from build123d import *

# Parameters (mm, degrees)
SKETCH2_W           = 5
SKETCH2_H           = 5.6
SKETCH2_R           = 1.5
BOSS_EXTRUDE1_DEPTH = 3
SKETCH5_W           = 5
SKETCH5_H           = 8
BOSS_EXTRUDE4_DEPTH = 3
BOSS_EXTRUDE5_DEPTH = 5
FILLET3_R           = 1


with BuildPart() as part:
    # Sketch2 → Boss-Extrude1 (new body)
    # profile 1 of 3: a face of its own
    with BuildSketch(Plane.XY):
        with Locations((-5, 0)):
            Rectangle(SKETCH2_W, SKETCH2_H)
        with Locations((-5, 0)):
            Circle(SKETCH2_R, mode=Mode.SUBTRACT)
    # profile 2 of 3: a face of its own
    with BuildSketch(Plane.XY):
        Rectangle(SKETCH2_W, SKETCH2_H)
    # profile 3 of 3: a face of its own
    with BuildSketch(Plane.XY):
        with Locations((5, 0)):
            Rectangle(SKETCH2_W, SKETCH2_H)
        with Locations((5, 0)):
            Circle(SKETCH2_R, mode=Mode.SUBTRACT)
    extrude(amount=BOSS_EXTRUDE1_DEPTH)

    # Sketch5 → Boss-Extrude4 (add)
    with BuildSketch(Plane.XY.offset(3)):
        with Locations((0, 6.8)):
            Rectangle(SKETCH5_W, SKETCH5_H)
    extrude(amount=-BOSS_EXTRUDE4_DEPTH)

    # Sketch6 → Boss-Extrude5 (add)
    with BuildSketch(Plane(origin=(2.5, 0, 0), x_dir=(0, 0, -1), z_dir=(1, 0, 0))):
        Polygon((0, 5.8), (11, 11.8), (11, 15.8), (-3, 12.8), (-3, 10.8), (0, 10.8), align=None)
    extrude(amount=-BOSS_EXTRUDE5_DEPTH)

    # Fillet3
    fillet3_edges = [part.edges().sort_by_distance(p)[0] for p in [
        (0, -2.8, 3),
        (-7.5, -2.8, 1.5),
        (-7.5, 2.8, 1.5),
        (7.5, 2.8, 1.5),
        (7.5, -2.8, 1.5),
        (7.5, 0, 3),
        (-5, 2.8, 3),
        (5, 2.8, 3),
        (-2.5, 7.8, 3),
        (2.5, 7.8, 3),
        (-2.5, 4.3, 0),
        (-7.5, 0, 3),
        (2.5, 4.3, 0),
        (2.5, 8.8, -5.5),
        (2.5, 13.8, -11),
        (2.5, 14.3, -4),
        (-2.5, 8.8, -5.5),
        (0, 11.8, -11),
        (-2.5, 13.8, -11),
        (-2.5, 14.3, -4),
        (0, 12.8, 3),
        (0, 5.8, 0),
    ]]
    fillet(fillet3_edges, radius=FILLET3_R - 0.0001)  # a hair under: the kernel refuses the full size


solid = part.part
Here's how the part is built. I have some questions about the finished solid (model axes, mm). A direction names the side the tool comes from. Coordinates: 2 decimals unless noted, no trailing zeros. Order: outer loops, then holes, each group sorted by start corner. A loop starts at its lowest first (then second) coordinate and runs counter-clockwise, first axis right, second up. Notation, with made-up numbers: M 23,62.25 L 27,62.25 A26 cw 27,87.25 Z; hole C 37,-26 d8. An arc over 180 degrees is marked long. Answer as CSV lines item,"result". Start each with the question number.
1. I need wall thicknesses on line 1 (Y direction, x = 5, z = 1.1); line 2 (Z direction, x = 2, y = -0.25); line 3 (X direction, y = 5.5, z = 1.5). Which ranges of each line are inside material? Lowest first, please. Write a range as [from, to].
2. I want a section at B-B, the plane y = 0. Count the separate pieces of the cut face and the enclosed holes in it, and give its area (3 significant figures).
3. I want a section at C-C, the plane x = -0.75. Write out the boundary of the cut face in (y, z).
4. I want a section at A-A, the plane x = 5. Write out the boundary of the cut face in (y, z).
5. I want a section at D-D, the plane y = 4.75. Write out the boundary of the cut face in (x, z), and give its area (3 significant figures).
6. On a 3-axis mill with a long thin cutter (end or side, diameter ignored), from which of +Z, -Z, +X, -X, +Y, -Y can I reach the whole of each face in a straight line? I mean faces 1 (the flat face through (2.5, 10, -3)), 2 (the cylindrical face through (7.215, 0.025, 2.699)). Say none if no direction works.
7. For pin 1 (8 mm diameter, centred on x = 2.5, y = 13, fed in from -Z); pin 2 (9 mm diameter, centred on x = 3.5, y = 2, fed in from -Z); pin 3 (3 mm diameter, centred on x = -1.5, z = -0.5, fed in from +Y); pin 4 (6 mm diameter, centred on y = 7, z = -3.5, fed in from +X), each with a flat end and sliding along its axis, tell me the tip position at first contact or that it passes through.
8. We'd pull the mould along Y, two halves only. Please class faces 3 (the cylindrical face through (-7.199, 2.515, 1.014)), 4 (the cylindrical face through (2.215, 4.02, 0.301)), 5 (the flat face through (0, -2.8, 1)), 6 (the cylindrical face through (-2.215, 6.967, 2.699)): released by +Y, released by -Y, zero draft, split by the parting line, or undercut.
Recorded:
1,line 1,"y = [-2.8, -1.5], [1.5, 2.8]"
1,line 2,"z = [0, 3]"
1,line 3,"x = [-2.5, 2.5]"
2,separate pieces,"3"
2,enclosed holes,"0"
2,area,"26.6 mm2"
3,outline,"M -2.8,0 L 5.21,0 A1 cw 6.08,-0.52 L 11.52,-10.48 A1 ccw 12.39,-11 L 15.8,-11 L 12.97,2.21 A1 ccw 11.99,3 L -1.8,3 A1 ccw -2.8,2 Z"
4,outline,"M -2.8,0 L -1.5,0 L -1.5,3 L -1.8,3 A1 ccw -2.8,2 Z; M 1.5,0 L 2.8,0 L 2.8,2 A1 ccw 1.8,3 L 1.5,3 Z"
5,outline,"M -2.5,1 A1 ccw -1.5,0 L 1.5,0 A1 ccw 2.5,1 L 2.5,2 A1 ccw 1.5,3 L -1.5,3 A1 ccw -2.5,2 Z"
5,area,"14.1 mm2"
6,face 1,"+Z, -Z, +X, +Y"
6,face 2,"+Z, +X, +Y, -Y"
7,pin 1,"stops at z = -11"
7,pin 2,"stops at z = -0.58"
7,pin 3,"stops at y = 13.87"
7,pin 4,"stops at x = 2.5"
8,face 3,"released by +Y"
8,face 4,"undercut"
8,face 5,"released by -Y"
8,face 6,"zero draft"
